CAD build for the part. Positions are in the model's coordinates, mm. Coordinates: 2 decimals unless noted, no trailing zeros. Write each loop counter-clockwise with the first axis right and the second up, starting at its lowest first coordinate (ties: lowest second). Pieces come first, ordered by that corner, then holes. Notation, with made-up numbers: (75.25, 9.5) - (99.25, 9.5) arc R12 cw to (99.25, 19.5) - close; hole circle Ø6 at (38.25, 13). An arc over 180 degrees is marked (long way). One line per question, with ' | ' between items. Start each with the question number.
1. Flat gauge pins, fed straight in: P1, Ø5, axis at y = 7, z = -0.5, coming from the +X side; P2, Ø5, axis at y = 2.5, z = -13, coming from the +X side; P3, Ø4, axis at y = 5.5, z = -20, coming from the +X side; P4, Ø2, axis at y = 8, z = 2, coming from the -X side. Where does each tip first touch, or does it go through?
2. Two-plate mould, pull along Z, no slides. Class faces 1 (the cylindrical face through (-1.08, 4.93, -17.12)), 2 (the cylindrical face through (-52.45, 4.93, 4.75)), 3 (the cylindrical face through (-107.53, 4.93, 23.58)): +Z half, -Z half, draft (parallel to the pull), parting line (faces both ways), or undercut.
3. Band-saw the part on A-A, the plane x = 0. Give the number of separate pieces and of enclosed holes in the cut face, then the cut area to 3 significant figures.
4. Probe line 1 (Z direction, x = 0, y = 4.5); line 2 (Z direction, x = -0.5, y = 8.75); line 3 (X direction, y = 5, z = 0). List the from-to ranges inside material, lowest first.
5. Band-saw the part on D-D, the plane x = -50.5. Write the cut outline in (y, z).
6. Band-saw the part on B-B, the plane z = -11.5. Write the cut outline in (x, y).
from build123d import *

# Parameters (mm, degrees)
SKETCH1_R           = 5
BOSS_EXTRUDE1_DEPTH = 10
FILLET1_R           = 10


with BuildPart() as part:
    # Sketch1 → Boss-Extrude1 (new body)
    with BuildSketch(Plane(origin=(0, 0, 0), x_dir=(1, 0, 0), z_dir=(0, 1, 0))):
        with BuildLine():
            ThreePointArc((10.228609777, 26.046670488), (6.184117748, 31.09707028), (0, 33))
            ThreePointArc((0, 33), (-57.565554835, 21.913887087), (-106.896551724, -9.75862069))
            ThreePointArc((-106.896551724, -9.75862069), (-107.383655881, -23.74400666), (-93.411472897, -24.522719629))
            ThreePointArc((-93.411472897, -24.522719629), (-50.8758669, -4.476742461), (-4.17684665, -9.983146536))
            ThreePointArc((-4.17684665, -9.983146536), (4.753191306, -9.721956341), (10.443773705, -2.834934477))
            ThreePointArc((10.443773705, -2.834934477), (5.699126861, 11.571322519), (10.228609777, 26.046670488))
        make_face()
        Circle(SKETCH1_R, mode=Mode.SUBTRACT)
        with Locations((0, 22)):
            Circle(SKETCH1_R, mode=Mode.SUBTRACT)
    extrude(amount=BOSS_EXTRUDE1_DEPTH)

    # Fillet1
    fillet1_edges = [part.edges().sort_by_distance(p)[0] for p in [
        (10.443773705, 5, 2.834934477),
        (10.228609777, 5, -26.046670488),
    ]]
    fillet(fillet1_edges, radius=FILLET1_R)


solid = part.part
Filled in:
1) P1: stops at x = 7.73 | P2: stops at x = 5.98 | P3: stops at x = 7.51 | P4: stops at x = -99.32
2) face 1: undercut | face 2: +Z half | face 3: parting line
3) separate pieces: 3 | enclosed holes: 0 | area: 224 mm²
4) line 1: z = -32.68 to -27, -17 to -5, 5 to 9.71 | line 2: z = -32.79 to -26.97, -17.03 to -4.97, 4.97 to 9.81 | line 3: x = -95.61 to -5, 5 to 7.73
5) outline: (0, -24.54) - (10, -24.54) - (10, 4.42) - (0, 4.42) - close
6) outline: (-78.76, 0) - (5.7, 0) - (5.7, 10) - (-78.76, 10) - close
